from build123d import *

# Parameters (mm, degrees)
F0_R     = 10.9
F1_DEPTH = 6.35


with BuildPart() as f1:
    # F0 (on Front) → F1 (new body)
    with BuildSketch(Plane.XZ):
        with BuildLine():
            ThreePointArc((11.341128, 43.011204), (12.355613, 45.78938), (12.7, 48.726868))
            ThreePointArc((12.7, 48.726868), (-2.937488, 61.082481), (-11.341128, 43.011204))
            ThreePointArc((-11.341128, 43.011204), (-10.922306, 42.315719), (-10.519233, 41.610989))
            ThreePointArc((-10.519233, 41.610989), (0, 36.026868), (10.519233, 41.610989))
            ThreePointArc((10.519233, 41.610989), (10.922306, 42.315719), (11.341128, 43.011204))
        make_face()
        Polygon((0, 59.49445), (9.325, 54.110659), (9.325, 43.343077), (0, 37.959285), (-9.325, 43.343077), (-9.325, 54.110659), align=None, mode=Mode.SUBTRACT)
        with BuildLine():
            ThreePointArc((-10.519233, 41.610989), (-10.922306, 42.315719), (-11.341128, 43.011204))
            ThreePointArc((-11.341128, 43.011204), (-10.95258, 42.297949), (-10.519233, 41.610989))
        make_face()
        with BuildLine():
            ThreePointArc((10.519233, 41.610989), (10.95258, 42.297949), (11.341128, 43.011204))
            ThreePointArc((11.341128, 43.011204), (10.922306, 42.315719), (10.519233, 41.610989))
        make_face()
        with BuildLine():
            ThreePointArc((10.519233, 41.610989), (0, 36.026868), (-10.519233, 41.610989))
            ThreePointArc((-10.519233, 41.610989), (-5.967201, 23.149777), (-11.428743, 4.936899))
            ThreePointArc((-11.428743, 4.936899), (-24.300415, -7.383263), (-41.497408, -12.044784))
            ThreePointArc((-41.497408, -12.044784), (-33.106319, -16.057504), (-29.700323, -24.712646))
            ThreePointArc((-29.700323, -24.712646), (-30.023908, -27.561217), (-30.978175, -30.26463))
            ThreePointArc((-30.978175, -30.26463), (-17.266312, -17.091848), (1.237274, -12.715244))
            ThreePointArc((1.237274, -12.715244), (18.342683, -17.702358), (30.978175, -30.26463))
            ThreePointArc((30.978175, -30.26463), (31.401801, -18.362646), (41.497408, -12.044784))
            ThreePointArc((41.497408, -12.044784), (24.300415, -7.383263), (11.428743, 4.936899))
            ThreePointArc((11.428743, 4.936899), (5.967201, 23.149777), (10.519233, 41.610989))
        make_face()
        Circle(F0_R, mode=Mode.SUBTRACT)
        with BuildLine():
            ThreePointArc((-29.700323, -24.712646), (-33.106319, -16.057504), (-41.497408, -12.044784))
            ThreePointArc((-41.497408, -12.044784), (-42.309258, -12.048077), (-43.120978, -12.033109))
            ThreePointArc((-43.120978, -12.033109), (-53.398846, -31.062646), (-31.779849, -31.67652))
            ThreePointArc((-31.779849, -31.67652), (-31.386952, -30.966066), (-30.978175, -30.26463))
            ThreePointArc((-30.978175, -30.26463), (-30.023908, -27.561217), (-29.700323, -24.712646))
        make_face()
        Polygon((-51.725323, -19.328855), (-42.400323, -13.945064), (-33.075323, -19.328855), (-33.075323, -30.096438), (-42.400323, -35.480229), (-51.725323, -30.096438), align=None, mode=Mode.SUBTRACT)
        with BuildLine():
            ThreePointArc((-43.120978, -12.033109), (-42.309258, -12.048077), (-41.497408, -12.044784))
            ThreePointArc((-41.497408, -12.044784), (-42.309006, -12.012975), (-43.120978, -12.033109))
        make_face()
        with BuildLine():
            ThreePointArc((43.120978, -12.033109), (42.309006, -12.012975), (41.497408, -12.044784))
            ThreePointArc((41.497408, -12.044784), (42.309258, -12.048077), (43.120978, -12.033109))
        make_face()
        with BuildLine():
            ThreePointArc((43.120978, -12.033109), (42.309258, -12.048077), (41.497408, -12.044784))
            ThreePointArc((41.497408, -12.044784), (31.401801, -18.362646), (30.978175, -30.26463))
            ThreePointArc((30.978175, -30.26463), (31.386952, -30.966066), (31.779849, -31.67652))
            ThreePointArc((31.779849, -31.67652), (46.03419, -36.881665), (55.100323, -24.712646))
            ThreePointArc((55.100323, -24.712646), (51.631854, -15.990901), (43.120978, -12.033109))
        make_face()
        Polygon((42.400323, -35.480229), (33.075323, -30.096438), (33.075323, -19.328855), (42.400323, -13.945064), (51.725323, -19.328855), (51.725323, -30.096438), align=None, mode=Mode.SUBTRACT)
        with BuildLine():
            ThreePointArc((31.779849, -31.67652), (31.386952, -30.966066), (30.978175, -30.26463))
            ThreePointArc((30.978175, -30.26463), (31.356426, -30.983399), (31.779849, -31.67652))
        make_face()
        with BuildLine():
            ThreePointArc((-30.978175, -30.26463), (-31.386952, -30.966066), (-31.779849, -31.67652))
            ThreePointArc((-31.779849, -31.67652), (-31.356426, -30.983399), (-30.978175, -30.26463))
        make_face()
    extrude(amount=F1_DEPTH)


solid = f1.part
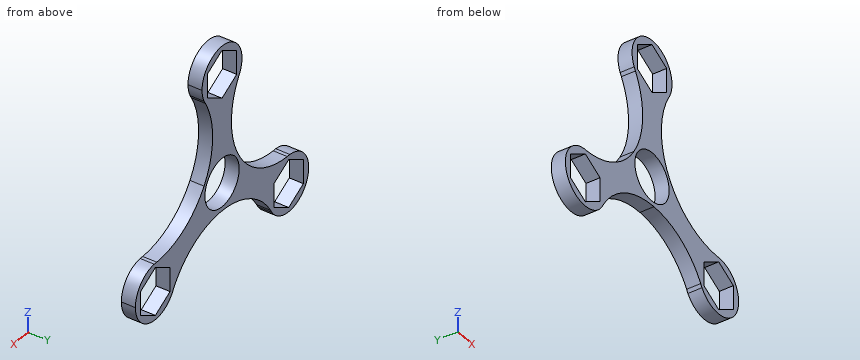
Geometry check sheet. Reference: the model listing, model coordinates, mm. Give positions to 0.01 mm unless a question says otherwise; leave off trailing zeros. Loops run counter-clockwise (first coordinate to the right, second up) from the corner with the lowest first, then second, coordinate; pieces in that order, holes last. Notation, with made-up numbers: M 31,-19 L 42,-19 A15 ccw 42,-7 Z; hole C 71.5,-11 d4. An arc over 180 degrees is marked long. Write each question's results on one line, items separated by ' | '.
1) Gauge pin test, flat ends, axial feed: pin 1 (10 mm diameter, centred on x = 36.5, z = -26, fed in from +Y); pin 2 (3 mm diameter, centred on y = -2, z = -26.5, fed in from +X); pin 3 (1 mm diameter, centred on x = 21, y = -2, fed in from +Z); pin 4 (3 mm diameter, centred on y = -3, z = -26.5, fed in from -X). Record the tip position at first contact, or that the pin passes through.
Answers follow:
pin 1: y = 0 | pin 2: x = 55.1 | pin 3: z = -4.91 | pin 4: x = -55.1
2) Section check D-D, the plane y = -3. Count the separate pieces of the cut face and the enclosed holes in it, plus the area to 3 significant figures.
Answers follow:
separate pieces: 1 | enclosed holes: 4 | area: 1,800 mm2
3) Section check A-A, the plane x = -1.5. Record the boundary of the cut face in (y, z), plus the area to 3 significant figures.
Answers follow:
outline: M -6.35,-12.73 L 0,-12.73 L 0,-10.8 L -6.35,-10.8 Z; M -6.35,10.8 L 0,10.8 L 0,38.83 L -6.35,38.83 Z; M -6.35,58.63 L 0,58.63 L 0,61.34 L -6.35,61.34 Z | area: 207 mm2
4) Section check B-B, the plane z = 50.5. Record the boundary of the cut face in (x, y) (3 decimals), plus the area to 3 significant figures.
Answers follow:
outline: M -12.576,-6.35 L -9.325,-6.35 L -9.325,0 L -12.576,0 Z; M 9.325,-6.35 L 12.576,-6.35 L 12.576,0 L 9.325,0 Z | area: 41.3 mm2
5) Section check C-C, the plane x = -34.5. Record the boundary of the cut face in (y, z), plus the area to 3 significant figures.
Answers follow:
outline: M -6.35,-34.66 L 0,-34.66 L 0,-30.92 L -6.35,-30.92 Z; M -6.35,-18.51 L 0,-18.51 L 0,-11.25 L -6.35,-11.25 Z | area: 69.8 mm2
6) Thickness scan on line 1 (Z direction, x = 0, y = -4.75); line 2 (Z direction, x = -2.5, y = -2.25); line 3 (X direction, y = -2, z = -29). Record the ranges inside material, lowest first.
Answers follow:
line 1: -12.69 to -10.9, 10.9 to 37.96, 59.49 to 61.43 | line 2: -12.78 to -10.61, 10.61 to 39.4, 58.05 to 61.18 | line 3: -54.35 to -51.73, -33.08 to -30.19, 30.19 to 33.08, 51.73 to 54.35
